The model under review builds one solid part; all positions refer to its coordinate system, in mm. Face numbers are marked on the shaded views. A direction names the side the tool comes from. Coordinates: 2 decimals unless noted, no trailing zeros. Order: outer loops, then holes, each group sorted by start corner. A loop starts at its lowest first (then second) coordinate and runs counter-clockwise, first axis right, second up. Notation, with made-up numbers: M -18.75,15 L 3.25,15 A15 cw 3.25,28 Z; hole C 88.25,9.5 d8. An arc over 180 degrees is marked long. Answer in a Markdown table with one row per item.
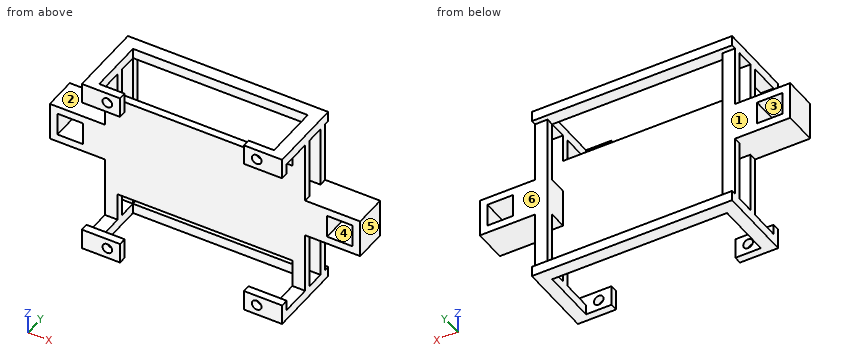
from build123d import *

# Parameters (mm, degrees)
SKETCH1_W             = 5
SKETCH1_H             = 63
BOSS_EXTRUDE1_DEPTH   = 3
BOSS_EXTRUDE1_2_DEPTH = 3
SKETCH3_W             = 78.71
SKETCH3_H             = 5
BOSS_EXTRUDE3_DEPTH   = 4
SKETCH4_W             = 78.71
SKETCH4_H             = 5
BOSS_EXTRUDE4_DEPTH   = 4
SKETCH6_W             = 15
SKETCH6_H             = 3
BOSS_EXTRUDE5_DEPTH   = 5.645
SKETCH7_W             = 16
SKETCH7_H             = 15
SKETCH7_W_2           = 10
SKETCH7_H_2           = 9
BOSS_EXTRUDE6_DEPTH   = 3
SKETCH5_W             = 5
SKETCH5_H             = 4
LEGS_DEPTH            = 25
SKETCH12_W            = 15
SKETCH12_H            = 8
SKETCH12_R            = 1.905
BOSS_EXTRUDE10_DEPTH  = 3
SKETCH13_W            = 21.645
SKETCH13_H            = 15
SKETCH13_W_2          = 10
SKETCH13_H_2          = 9
COPY_2_DEPTH          = 3
BOSS_EXTRUDE11_DEPTH  = 3
SKETCH15_W            = 10
SKETCH15_H            = 9
BOSS_EXTRUDE12_DEPTH  = 10


with BuildPart() as part:
    # Sketch1 → Boss-Extrude1 (new body)
    with BuildSketch(Plane(origin=(0, 0, 0), x_dir=(1, 0, 0), z_dir=(0, 1, 0))):
        with Locations((-36.855, 0)):
            Rectangle(SKETCH1_W, SKETCH1_H)
    extrude(amount=BOSS_EXTRUDE1_DEPTH)



with BuildPart() as body_2:
    # Sketch1 → Boss-Extrude1 2 (new body)
    with BuildSketch(Plane(origin=(0, 0, 0), x_dir=(1, 0, 0), z_dir=(0, 1, 0))):
        with Locations((36.855, 0)):
            Rectangle(SKETCH1_W, SKETCH1_H)
    extrude(amount=BOSS_EXTRUDE1_2_DEPTH)


with BuildPart() as part_1:
    add(part.part)

    add(body_2.part)  # Boss-Extrude3 merges body 2
    # Sketch3 → Boss-Extrude3 (add)
    with BuildSketch(Plane.XY.offset(31.5)):
        with Locations((0, 2.5)):
            Rectangle(SKETCH3_W, SKETCH3_H)
    extrude(amount=BOSS_EXTRUDE3_DEPTH)

    # Sketch4 → Boss-Extrude4 (add)
    with BuildSketch(Plane(origin=(0, 0, -31.5), x_dir=(-1, 0, 0), z_dir=(0, 0, -1))):
        with Locations((0, 2.5)):
            Rectangle(SKETCH4_W, SKETCH4_H)
    extrude(amount=BOSS_EXTRUDE4_DEPTH)

    # Sketch6 → Boss-Extrude5 (add)
    with BuildSketch(Plane.ZY.offset(39.355)):
        with Locations((0, 1.5)):
            Rectangle(SKETCH6_W, SKETCH6_H)
    extrude(amount=BOSS_EXTRUDE5_DEPTH)

    # Sketch7 → Boss-Extrude6 (add)
    with BuildSketch(Plane(origin=(0, 3, 0), x_dir=(1, 0, 0), z_dir=(0, 1, 0))):
        with Locations((-53, 0)):
            Rectangle(SKETCH7_W, SKETCH7_H)
        with Locations((-53, 0)):
            Rectangle(SKETCH7_W_2, SKETCH7_H_2, mode=Mode.SUBTRACT)
    extrude(amount=-BOSS_EXTRUDE6_DEPTH)

    # Sketch5 → legs (add)
    with BuildSketch(Plane.XZ):
        with Locations((-36.855, 33.5)):
            Rectangle(SKETCH5_W, SKETCH5_H)
        with Locations((36.855, 33.5)):
            Rectangle(SKETCH5_W, SKETCH5_H)
        with Locations((-36.855, -33.5)):
            Rectangle(SKETCH5_W, SKETCH5_H)
        with Locations((36.855, -33.5)):
            Rectangle(SKETCH5_W, SKETCH5_H)
    extrude(amount=LEGS_DEPTH)

    # Sketch12 → Boss-Extrude10 (add)
    # profile 1 of 4: a face of its own
    with BuildSketch(Plane.XZ.offset(25)):
        with Locations((31.855, 31.5)):
            Rectangle(SKETCH12_W, SKETCH12_H)
        with Locations(Location((29.355, 31.5, 0), (0, 0, 270))):
            Circle(SKETCH12_R, mode=Mode.SUBTRACT)
    # profile 2 of 4: a face of its own
    with BuildSketch(Plane.XZ.offset(25)):
        with Locations((31.855, -31.5)):
            Rectangle(SKETCH12_W, SKETCH12_H)
        with Locations(Location((29.355, -31.5, 0), (0, 0, 90))):
            Circle(SKETCH12_R, mode=Mode.SUBTRACT)
    # profile 3 of 4: a face of its own
    with BuildSketch(Plane.XZ.offset(25)):
        with Locations((-31.855, -31.5)):
            Rectangle(SKETCH12_W, SKETCH12_H)
        with Locations(Location((-29.355, -31.5, 0), (0, 0, 270))):
            Circle(SKETCH12_R, mode=Mode.SUBTRACT)
    # profile 4 of 4: a face of its own
    with BuildSketch(Plane.XZ.offset(25)):
        with Locations((-31.855, 31.5)):
            Rectangle(SKETCH12_W, SKETCH12_H)
        with Locations(Location((-29.355, 31.5, 0), (0, 0, 90))):
            Circle(SKETCH12_R, mode=Mode.SUBTRACT)
    extrude(amount=-BOSS_EXTRUDE10_DEPTH)

    # Sketch13 → copy 2 (add)
    with BuildSketch(Plane(origin=(0, 3, 0), x_dir=(1, 0, 0), z_dir=(0, 1, 0))):
        with Locations((50.1775, 0)):
            Rectangle(SKETCH13_W, SKETCH13_H)
        with Locations((53, 0)):
            Rectangle(SKETCH13_W_2, SKETCH13_H_2, mode=Mode.SUBTRACT)
    extrude(amount=-COPY_2_DEPTH)

    # Sketch14 → Boss-Extrude11 (add)
    with BuildSketch(Plane(origin=(0, -10, 0), x_dir=(-1, 0, 0), z_dir=(0, -1, 0))):
        Polygon((-39.355, 35.5), (-34.355, 35.5), (-34.355, 20.5), (34.355, 20.5), (34.355, 35.5), (39.355, 35.5), (39.355, -35.5), (34.355, -35.5), (34.355, -20.5), (-34.355, -20.5), (-34.355, -35.5), (-39.355, -35.5), align=None)
    extrude(amount=-BOSS_EXTRUDE11_DEPTH)

    # Sketch15 → Boss-Extrude12 (add)
    # profile 1 of 2: a face of its own
    with BuildSketch(Plane.XZ):
        Polygon((-61, 7.5), (-61, -7.5), (-39.355, -7.5), (-34.355, -7.5), (-34.355, 7.5), (-39.355, 7.5), align=None)
        with Locations((-53, 0)):
            Rectangle(SKETCH15_W, SKETCH15_H, mode=Mode.SUBTRACT)
    # profile 2 of 2: a face of its own
    with BuildSketch(Plane.XZ):
        Polygon((34.355, -7.5), (34.355, 7.5), (39.355, 7.5), (61, 7.5), (61, -7.5), (39.355, -7.5), align=None)
        with Locations((53, 0)):
            Rectangle(SKETCH15_W, SKETCH15_H, mode=Mode.SUBTRACT)
    extrude(amount=BOSS_EXTRUDE12_DEPTH)


solid = part_1.part
(1) Machinability: for the marked faces 1, 2 and 3, which of the approach directions +Z, -Z, +X, -X, +Y, -Y give a long, thin tool a straight path to every point of the face, cutting with its end or side? Answer none if there is none.
Report:
| item | result |
|---|---|
| face 1 | +X, -X, +Y |
| face 2 | -X |
| face 3 | +Y, -Y |
(2) Take a section at C-C (x = -52.5). Write out the cut boundary in (y, z).
Report:
| item | result |
|---|---|
| outline | M -10,-7.5 L 3,-7.5 L 3,-4.5 L -10,-4.5 Z; M -10,4.5 L 3,4.5 L 3,7.5 L -10,7.5 Z |
(3) Take a section at A-A (x = -7). Write out the cut boundary in (y, z), then the cut area to 3 significant figures.
Report:
| item | result |
|---|---|
| outline | M -10,-20.5 L -7,-20.5 L -7,20.5 L -10,20.5 Z; M 0,-35.5 L 5,-35.5 L 5,-31.5 L 0,-31.5 Z; M 0,31.5 L 5,31.5 L 5,35.5 L 0,35.5 Z |
| area | 163 mm^2 |
(4) Insertion check: P1, Ø4, axis at x = -36.5, z = -23.5, coming from the -Y side; P2, Ø0.9, axis at y = -23.5, z = 30.5, coming from the -X side (3 decimals); P3, Ø0.9, axis at y = -23, z = -30, coming from the +X side (3 decimals). Each pin has a flat end and moves straight along its axis. Give the tip position at first contact, or say it passes through.
Report:
| item | result |
|---|---|
| P1 | y = -10 |
| P2 | x = -39.355 |
| P3 | x = 39.355 |
(5) Take a section at B-B (y = -16.75). Write out the cut boundary in (x, z) (3 decimals), then the cut area to 3 significant figures.
Report:
| item | result |
|---|---|
| outline | M -39.355,-35.5 L -34.355,-35.5 L -34.355,-31.5 L -39.355,-31.5 Z; M -39.355,31.5 L -34.355,31.5 L -34.355,35.5 L -39.355,35.5 Z; M 34.355,-35.5 L 39.355,-35.5 L 39.355,-31.5 L 34.355,-31.5 Z; M 34.355,31.5 L 39.355,31.5 L 39.355,35.5 L 34.355,35.5 Z |
| area | 80.0 mm^2 |
(6) To check wall thickness, follow line 1 (X direction, y = -23.8, z = -31.5) (3 decimals); line 2 (Y direction, x = 38.5, z = -23.5); line 3 (X direction, y = 2.25, z = 1) (3 decimals). State the ranges of each line that lie inside material, in increasing order. Write a range as [from, to].
Report:
| item | result |
|---|---|
| line 1 | [-39.355, -31.26], [-27.45, -24.355], [24.355, 27.45], [31.26, 39.355] |
| line 2 | [-10, -7], [0, 3] |
| line 3 | [-61, -58], [-48, -34.355], [34.355, 48], [58, 61] |
(7) The part is to be moulded in two halves that separate along X. For the marked faces 4, 5 and 6, say which applies: +X half, -X half, draft (parallel to the pull), parting line (faces both ways), or undercut.
Report:
| item | result |
|---|---|
| face 4 | undercut |
| face 5 | +X half |
| face 6 | draft |
